Here's how the part is built. I have some questions about the finished solid (model axes, mm). Face numbers are marked on the shaded views. A direction names the side the tool comes from. Coordinates: 2 decimals unless noted, no trailing zeros. Loops run counter-clockwise (first coordinate to the right, second up) from the corner with the lowest first, then second, coordinate; pieces in that order, holes last. Notation, with made-up numbers: (-0.75, 81.5) -> (25.25, 81.5) arc R21 ccw to (25.25, 87.5) -> close; hole circle Ø2 at (38, 83.5). An arc over 180 degrees is marked (long way). Use CSV: the item, a comma, the result in double quotes. Start each with the question number.
from build123d import *

# Parameters (mm, degrees)
F0_W      = 43.5
F0_H      = 20
F1_DEPTH  = 21
F2_W      = 23.5
F2_H      = 2
F3_DEPTH  = 79
F4_W      = 8.7595684454
F4_H      = 3.4760199487
F4_W_2    = 14.3907200545
F4_H_2    = 1.9311879296
F5_DEPTH  = 21.001
F6_W      = 18.0619247258
F6_H      = 11.0779828392
F7_DEPTH  = 20.001
F8_W      = 8.364611771
F8_H      = 3.2224319875
F9_DEPTH  = 43.501
F10_DEPTH = 13.8
F11_DEPTH = 16.0159093717
F12_W     = 5.3562937983
F12_H     = 8.364611771
F13_DEPTH = 3.3


# Not quite as in the source:
# - an extrude ends at something that could not be found from the text; its depth is read off the source's solid


with BuildPart() as f1:
    # F0 (on Front) → F1 (new body)
    with BuildSketch(Plane.XZ):
        with Locations((21.75, 10)):
            Rectangle(F0_W, F0_H)
    extrude(amount=F1_DEPTH)

    # F2 (on Front) → F3 (cut, through all)
    with BuildSketch(Plane.XZ):
        with Locations((15.8696506918, 1)):
            Rectangle(F2_W, F2_H)
    extrude(amount=-F3_DEPTH, mode=Mode.SUBTRACT)

    # F4 (on face) → F5 (cut, through all)
    with BuildSketch(Plane.XZ.offset(21)):
        Polygon((25.5898274481, 20), (9.7391782328, 20), (9.7391782328, 17.1561539173), (13.2151981816, 17.1561539173), (21.974766627, 17.1561539173), (25.5898274481, 17.1561539173), align=None)
        with Locations((17.5949824043, 15.418143943)):
            Rectangle(F4_W, F4_H)
        with Locations((15.9612530842, 0.9655939648)):
            Rectangle(F4_W_2, F4_H_2)
        Polygon((43.5, 20), (29.7610498965, 20), (29.7610498965, 15.5571838841), (43.5, 5.6157684885), align=None)
    extrude(amount=-F5_DEPTH, mode=Mode.SUBTRACT)

    # F6 (on Top) → F7 (cut, through all)
    with BuildSketch(Plane.XY):
        with Locations((38.8933513314, -10.4759179521)):
            Rectangle(F6_W, F6_H)
    extrude(amount=F7_DEPTH, mode=Mode.SUBTRACT)

    # F8 (on face) → F9 (cut, through all)
    with BuildSketch(Plane(origin=(0, 0, 0), x_dir=(0, -1, 0), z_dir=(-1, 0, 0))):
        with Locations((11.04275533, 14.9709172547)):
            Rectangle(F8_W, F8_H)
        Polygon((16.7677160352, 20), (4.9407021143, 20), (4.9407021143, 16.5821332484), (6.8604494445, 16.5821332484), (15.2250612155, 16.5821332484), (16.7677160352, 16.5821332484), align=None)
    extrude(amount=-F9_DEPTH, mode=Mode.SUBTRACT)

    # F10 (add): a face of the model
    f10_faces = [f1.faces().sort_by_distance(p)[0] for p in [
        (29.8623889685, -10.4104180179, 6.9700489552),
    ]]
    extrude(f10_faces, amount=F10_DEPTH)

    # F11 (cut, through all): a face of the model
    f11_faces = [f1.faces().sort_by_distance(p)[0] for p in [
        (39.1208034391, -16.0149093717, 12.034105167),
    ]]
    extrude(f11_faces, amount=-F11_DEPTH, mode=Mode.SUBTRACT)

    # F12 (on face) → F13 (join)
    with BuildSketch(Plane.XY.offset(13.3597012609)):
        with Locations((30.1198049788, -11.04275533)):
            Rectangle(F12_W, F12_H)
    extrude(amount=F13_DEPTH)


solid = f1.part
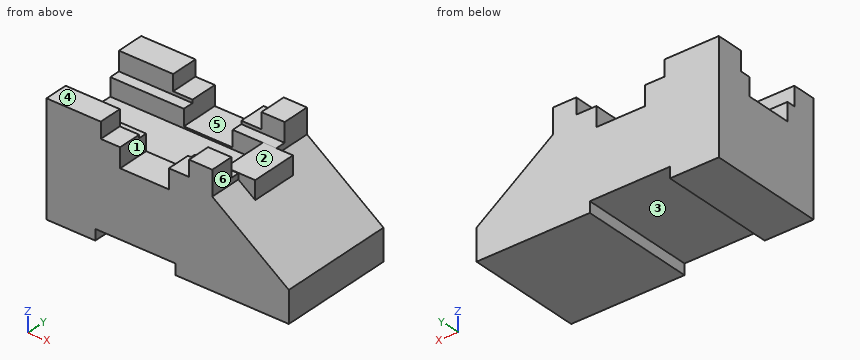
1) I want a section at B-B, the plane x = 12. Please give me the cut outline in (y, z).
2) Which directions (+Z, -Z, +X, -X, +Y, -Y) give clear straight access to the entire face, cutting with the end or side of a thin tool? Please do the marked faces 1, 2 and 3.
3) Thinking about a two-plate mould opening in X: for the marked faces 4, 5 and 6, which applies, pulls with the +X half, pulls with the -X half, needs draft (parallel to the pull), parting line crosses it, or undercut?
4) I want a section at A-A, the plane z = 17.75. Please give me the cut outline in (x, y), plus the area to 3 significant figures.
5) For P1, Ø1.5, axis at x = 20, y = -10.5, coming from the +Z side; P2, Ø3, axis at x = 24, y = -19.5, coming from the +Z side; P3, Ø1, axis at x = 31.5, z = 15.5, coming from the -Y side; P4, Ø1, axis at x = 24.5, z = 18, coming from the +Y side, each with a flat end and sliding along its axis, tell me the tip position at first contact or that it passes through.
6) Please list where these lines run through material, in increasing order: L1, parallel to Y at x = 12.5, z = 16.5; L2, parallel to Z at x = 16, y = -10.75; L3, parallel to Z at x = 33, y = -1.5. Write a range as [from, to].
7) I want a section at C-C, the plane y = -8.75. Please give me the cut outline in (x, z).
8) I want a section at D-D, the plane x = 20.5. Please give me the cut outline in (y, z), plus the area to 3 significant figures.
Return value:
1,outline,"(-21, 1.93) -> (0, 1.93) -> (0, 17.16) -> (-4.94, 17.16) -> (-4.94, 16.58) -> (-6.86, 16.58) -> (-6.86, 13.36) -> (-15.23, 13.36) -> (-15.23, 16.58) -> (-16.77, 16.58) -> (-16.77, 17.16) -> (-21, 17.16) -> close"
2,face 1,"+Z, +Y, -Y"
2,face 2,"+Z, +X, -X"
2,face 3,"-Z, +Y, -Y"
3,face 4,"needs draft"
3,face 5,"undercut"
3,face 6,"pulls with the +X half"
4,outline,"(0, -21) -> (9.74, -21) -> (9.74, -16.77) -> (0, -16.77) -> close; (0, -4.94) -> (9.74, -4.94) -> (9.74, 0) -> (0, 0) -> close; (25.59, -21) -> (29.76, -21) -> (29.76, -16.77) -> (25.59, -16.77) -> close; (25.59, -4.94) -> (29.76, -4.94) -> (29.76, 0) -> (25.59, 0) -> close"
4,area,"128 mm²"
5,P1,"stops at z = 13.36"
5,P2,"stops at z = 17.16"
5,P3,"stops at y = -15.23"
5,P4,"passes through"
6,L1,"y = [-21, -15.23], [-6.86, 0]"
6,L2,"z = [1.93, 13.36]"
6,L3,"z = [0, 13.21]"
7,outline,"(0, 0) -> (8.77, 0) -> (8.77, 1.93) -> (23.16, 1.93) -> (23.16, 0) -> (43.5, 0) -> (43.5, 5.62) -> (32.8, 13.36) -> (32.8, 16.66) -> (27.44, 16.66) -> (27.44, 13.36) -> (0, 13.36) -> close"
8,outline,"(-21, 1.93) -> (0, 1.93) -> (0, 13.68) -> (-6.86, 13.68) -> (-6.86, 13.36) -> (-15.23, 13.36) -> (-15.23, 13.68) -> (-21, 13.68) -> close"
8,area,"244 mm²"
